Autodesk Inventor part; units mm, degrees
ref_plane "Work Plane1" through (0, 0, -10) normal (0, 0, -1) x (-1, 0, 0)
ref_plane "Work Plane2" through (0, 0, -5) normal (0, 0, 1) x (1, 0, 0)
ref_plane "YZ Plane" through (0, 0, 0) normal (1, 0, 0) x (0, 1, 0)
sketch "Sketch1" plane through (0, 0, 0) normal (0, 0, 1) x (1, 0, 0)
  point P0 (0, 0)
sketch "Sketch2" plane through (0, 0, 0) normal (0, 0, 1) x (1, 0, 0)
  line L0 (-15, 130) -> (15, 130)
  line L1 (15, 130) -> (15, 0)
  line L2 (15, 0) -> (-15, 0)
  line L3 (-15, 0) -> (-15, 130)
  point P0 (0, 0)
  point P1 (0, 0)
  dimension "d0" = 30
  dimension "d1" = 130
extrude "Extrusion1" add sketch "Sketch2" along normal blind 5
ref_plane "Work Plane1" through (0, 0, -10) normal (0, 0, -1) x (-1, 0, 0)
sketch "Sketch4" plane through (0, 0, -10) normal (0, 0, -1) x (-1, 0, 0)
  line L0 (-15, 0) -> (-15, 130)
  line L1 (15, 0) -> (-15, 0)
  line L2 (-15, 130) -> (15, 130)
  line L3 (15, 130) -> (15, 0)
  line L4 (15, 0) -> (-15, 0)
  line L5 (-15, 0) -> (-15, 130)
  point P0 (0, 0)
extrude "Extrusion3" add sketch "Sketch4" along normal blind 5
sketch "Sketch5" plane through (0, 0, -10) normal (0, 0, 1) x (1, 0, 0)
  line L0 (-15, 130) -> (-15, 0)
  line L1 (15, 130) -> (15, 0)
  line L2 (-15, 130) -> (15, 130)
  line L3 (15, 130) -> (15, 115)
  line L4 (15, 115) -> (-15, 115)
  line L5 (-15, 115) -> (-15, 130)
  point P0 (0, 0)
  point P1 (15, 130)
  dimension "d12" = 15
extrude "Extrusion4" add sketch "Sketch5" along normal blind 10
sketch "Sketch6" plane through (0, 0, -10) normal (0, 0, 1) x (1, 0, 0)
  circle A0 centre (0, 10) radius 2.5
  line L0 (-15, 0) -> (15, 0)
  point P0 (0, 0)
  dimension "d15" = 5
  dimension "d16" = 10
  dimension "d45" = 18.0278
extrude "Extrusion5" cut sketch "Sketch6" along normal blind 15 and the other way blind 5
ref_plane "Work Plane2" through (0, 0, -5) normal (0, 0, 1) x (1, 0, 0)
sketch "Sketch9" plane through (0, 0, 5) normal (0, 0, 1) x (1, 0, 0)
  line L0 (15, 130) -> (-15, 130)
  line L1 (15, 0) -> (15, 130)
  line L2 (0, 84.3715) -> (0, -83.7026)
  line L3 (-15, 0) -> (15, 0)
  line L4 (-15, 122.5) -> (15, 122.5)
  line L5 (-15, 115) -> (15, 115)
  circle A0 centre (0, 122.5) radius 6
  point P0 (0, 0)
  point P1 (0, 0)
  dimension "d41" = 7.5
  dimension "d42" = 12
  dimension "d46" = 15
  dimension "d47" = 45.6285
  dimension "d48" = 213.7026
extrude "Extrusion7" cut sketch "Sketch9" against normal blind 20
properties part number "pendel"
Geometry: final body of the model. Coordinates: model frame, mm. A direction names the side the tool comes from. Give positions to 0.01 mm unless a question says otherwise; leave off trailing zeros. Write each loop counter-clockwise with the first axis right and the second up, starting at its lowest first coordinate (ties: lowest second). Pieces come first, ordered by that corner, then holes. Notation, with made-up numbers: M -35,-31.75 L -22,-31.75 A12 cw -22,-27.75 Z; hole C 24.5,57 d7. An arc over 180 degrees is marked long. Answer in a Markdown table with one row per item. Add a question column.
(1) Section D-D on z = -2.75. Return loops of the section in (x, y).
(2) Section A-A on y = 10. Return loops of the section in (x, z).
(3) Section C-C on y = 122.5. Return loops of the section in (x, z), and give its area (3 significant figures).
(4) Reachability of faces 1 (the flat face through (0, 0, 2)), 2 (the flat face through (0, 115, -5)) from +Z, -Z, +X, -X, +Y, -Y: full face, straight path, thin tool, end or side. Return the list, or none.
(5) Section B-B on x = 0. Return loops of the section in (y, z).
(6) First-contact query: pin 1 (3 mm diameter, centred on x = 9, z = -5.5, fed in from -Y); pin 2 (4 mm diameter, centred on x = 0, y = 10, fed in from +Z). Flat tips, straight axial feed; report the tip coordinate or a pass-through.
(7) Ray query, line 1 (Y direction, x = 0, z = -13.2); line 2 (Z direction, x = 6.75, y = 113.5); line 3 (X direction, y = 122.5, z = -0.5). Return the intervals inside material, ascending.
(8) Mould query, pull axis Z, two halves, no side actions, for faces 3 (the flat face through (15, 66, -12)), 4 (the flat face through (0, 58, -10)), 5 (the flat face through (0, 66, -15)). Classes: +Z half, -Z half, draft (parallel to the pull), parting line (faces both ways), or undercut.
Result set:
| question | item | result |
|---|---|---|
| 1 | outline | M -15,115 L 15,115 L 15,130 L -15,130 Z; hole C 0,122.5 d12 |
| 2 | outline | M -15,-15 L -2.5,-15 L -2.5,-10 L -15,-10 Z; M -15,0 L -2.5,0 L -2.5,5 L -15,5 Z; M 2.5,-15 L 15,-15 L 15,-10 L 2.5,-10 Z; M 2.5,0 L 15,0 L 15,5 L 2.5,5 Z |
| 3 | outline | M -15,-15 L -6,-15 L -6,5 L -15,5 Z; M 6,-15 L 15,-15 L 15,5 L 6,5 Z |
| 3 | area | 360 mm^2 |
| 4 | face 1 | +Z, -Z, +X, -X, -Y |
| 4 | face 2 | +X, -X, -Y |
| 5 | outline | M 0,-15 L 7.5,-15 L 7.5,-10 L 0,-10 Z; M 0,0 L 7.5,0 L 7.5,5 L 0,5 Z; M 12.5,-15 L 116.5,-15 L 116.5,5 L 12.5,5 L 12.5,0 L 115,0 L 115,-10 L 12.5,-10 Z; M 128.5,-15 L 130,-15 L 130,5 L 128.5,5 Z |
| 6 | pin 1 | stops at y = 115 |
| 6 | pin 2 | passes through |
| 7 | line 1 | y = 0 to 7.5, 12.5 to 116.5, 128.5 to 130 |
| 7 | line 2 | z = -15 to -10, 0 to 5 |
| 7 | line 3 | x = -15 to -6, 6 to 15 |
| 8 | face 3 | draft |
| 8 | face 4 | undercut |
| 8 | face 5 | -Z half |
